Work out the finished part from the listing and answer in its coordinate system (mm). A direction names the side the tool comes from. Round coordinates to 2 decimals unless told otherwise and drop trailing zeros. Loops run counter-clockwise (first coordinate to the right, second up) from the corner with the lowest first, then second, coordinate; pieces in that order, holes last. Notation, with made-up numbers: M 66,70.25 L 117,70.25 A17 ccw 117,85.25 Z; hole C -34.5,-26 d5. An arc over 180 degrees is marked long. One line per item, written item: value.
```python
from build123d import *

# Parameters (mm, degrees)
F1_DEPTH        = 5.1562
F2_R            = 40.005
F2_R_2          = 1.397
F3_DEPTH        = 5.1572
F4_W            = 32.5247
F4_H            = 5.1562
F5_DEPTH        = 5.1572
F5_COPIES_COUNT = 6


# Not quite as in the source:
# - a pattern or mirror of a feature is missing from the dataset's text; its kind, count and spacing are read off the source's solid


with BuildPart() as f1:
    # F0 (on Front) → F1 (new body)
    with BuildSketch(Plane.XZ):
        with BuildLine():
            Line((137.8481502717, 12.7), (79.9225977639, 113.03))
            ThreePointArc((79.9225977639, 113.03), (70.6255525078, 122.3270452561), (57.9255525078, 125.73))
            Line((57.9255525078, 125.73), (-57.9255525078, 125.73))
            ThreePointArc((-57.9255525078, 125.73), (-70.6255525078, 122.3270452561), (-79.9225977639, 113.03))
            Line((-79.9225977639, 113.03), (-137.8481502717, 12.7))
            ThreePointArc((-137.8481502717, 12.7), (-141.2511050156, 0), (-137.8481502717, -12.7))
            Line((-137.8481502717, -12.7), (-79.9225977639, -113.03))
            ThreePointArc((-79.9225977639, -113.03), (-70.6255525078, -122.3270452561), (-57.9255525078, -125.73))
            Line((-57.9255525078, -125.73), (57.9255525078, -125.73))
            ThreePointArc((57.9255525078, -125.73), (70.6255525078, -122.3270452561), (79.9225977639, -113.03))
            Line((79.9225977639, -113.03), (137.8481502717, -12.7))
            ThreePointArc((137.8481502717, -12.7), (141.2511050156, 0), (137.8481502717, 12.7))
        make_face()
    extrude(amount=-F1_DEPTH)

    # F2 (on face) → F3 (cut, through all)
    with BuildSketch(Plane.XZ):
        Circle(F2_R)
        with Locations((0, 46.4947)):
            Circle(F2_R_2)
        with Locations((-46.4947, 0)):
            Circle(F2_R_2)
        with Locations((0, -46.4947)):
            Circle(F2_R_2)
        with Locations((46.4947, 0)):
            Circle(F2_R_2)
    extrude(amount=-F3_DEPTH, mode=Mode.SUBTRACT)

    # F4 (on face) → F5 (cut, through all)
    with BuildSketch(Plane.XZ):
        with Locations((-41.66235, 120.6119)):
            Rectangle(F4_W, F4_H)
        with Locations((41.66235, 120.6119)):
            Rectangle(F4_W, F4_H)
    f5 = extrude(amount=-F5_DEPTH, mode=Mode.SUBTRACT)

    # F5_copies: F5 ×6 about axis
    f5_copies_axis = Axis((0, 0, 0), (0, 1, 0))
    for i in range(1, F5_COPIES_COUNT):
        add(f5.rotate(f5_copies_axis, i * 360 / F5_COPIES_COUNT), mode=Mode.SUBTRACT)


solid = f1.part
```
1) The mould has two halves that part along Z. Classify faces 1 (the face through (-108.48, 2.54, 63.57)), 2 (the face through (-123.165, 2.542, 22.739)), 3 (the face through (-109.291, 2.542, -62.163)): +Z half, -Z half, draft (parallel to the pull), parting line (faces both ways), or undercut.
Check values:
face 1: +Z half
face 2: undercut
face 3: -Z half
2) Find section C-C (x = 15). Give the vertices of the cut face in (y, z), then the cut area to 3 significant figures.
Check values:
outline: M 0,-125.73 L 5.16,-125.73 L 5.16,-37.09 L 0,-37.09 Z; M 0,37.09 L 5.16,37.09 L 5.16,125.73 L 0,125.73 Z
area: 914 mm2
3) Each of these flat-tipped pins is pushed along its axis until it touches: pin 1 (1.5 mm diameter, centred on y = 1.5, z = 120.5, fed in from +X); pin 2 (1.5 mm diameter, centred on y = 3.5, z = -55.5, fed in from -X). Where does it stop, or does it pass through?
Check values:
pin 1: x = 74.3
pin 2: x = -113.57
4) For faces 4 (the face through (-33, 5.156, -26)), 5 (the face through (81.28, 2.54, 95.29)), determine the directions among +Z, -Z, +X, -X, +Y, -Y from which every point of the face is accessible in a straight line to the end or side of a thin tool.
Check values:
face 4: +Z, -Z, +X, -X, +Y
face 5: +Y, -Y
5) Find section A-A (x = -54). Give the vertices of the cut face in (y, z), then the cut area to 3 significant figures.
Check values:
outline: M 0,-125.73 L 5.16,-125.73 L 5.16,-123.19 L 0,-123.19 Z; M 0,-118.03 L 5.16,-118.03 L 5.16,118.03 L 0,118.03 Z; M 0,123.19 L 5.16,123.19 L 5.16,125.73 L 0,125.73 Z
area: 1,240 mm2
6) Find the intervals of material crossed by probe 1 along Z at (x, y) = (0, 4) (3 decimals); probe 2 along Z at (x, y) = (-129, 4.4); probe 3 along Z at (x, y) = (-117.5, 4), in increasing order. Write a range as from..to.
Check values:
probe 1: -125.73..-47.892, -45.098..-40.005, 40.005..45.098, 47.892..125.73
probe 2: -28.03..-22.95, -12.63..12.63, 22.95..28.03
probe 3: -47.94..-38.51, -32.55..32.55, 38.51..47.94
7) Find section B-B (z = -18). Give the vertices of the cut face in (x, y), then the cut area to 3 significant figures.
Check values:
outline: M -134.79,0 L -131.86,0 L -131.86,5.16 L -134.79,5.16 Z; M -125.9,0 L -35.73,0 L -35.73,5.16 L -125.9,5.16 Z; M 35.73,0 L 125.9,0 L 125.9,5.16 L 35.73,5.16 Z; M 131.86,0 L 134.79,0 L 134.79,5.16 L 131.86,5.16 Z
area: 960 mm2
8) Find section D-D (y = 3.55). Give the number of separate pieces and of enclosed holes in the cut face, then the cut area to 3 significant figures.
Check values:
separate pieces: 1
enclosed holes: 17
area: 47,500 mm2
